CAD build for the part. Positions are in the model's coordinates, mm. Give positions to 0.01 mm unless a question says otherwise; leave off trailing zeros. Order: outer loops, then holes, each group sorted by start corner. A loop starts at its lowest first (then second) coordinate and runs counter-clockwise, first axis right, second up. Notation, with made-up numbers: (-27.75, 43) -> (-22.75, 43) arc R21 ccw to (-22.75, 62) -> close; hole circle Ø3 at (23, -10). An arc over 180 degrees is marked (long way). Use one line per item in the form item = value. Start each with the question number.
1) Drop flat-ended pins along their axis: P1, Ø1, axis at x = 0, z = -3.5, coming from the -Y side; P2, Ø2, axis at y = -1, z = 1, coming from the +X side; P3, Ø1.5, axis at x = -1, y = -1.5, coming from the +Z side; P4, Ø2, axis at x = -1, y = 2.5, coming from the -Z side. Give the stop position or say it passes through.
2) Probe line 1 (Y direction, x = 1.45, z = -0.5); line 2 (Y direction, x = 0.25, z = -0.75); line 3 (Z direction, x = -0.8, y = -0.25). List the from-to ranges inside material, lowest first.
3) Mould opens along Z. For faces 1 (the face through (1.86, -2, 3)), 2 (the face through (1.461, -0.963, -4.334)), 3 (the face through (0, -3, 0)) say: pulls with the +Z half, pulls with the -Z half, needs draft (parallel to the pull), parting line crosses it, or undercut.
4) Cut at C-C, the plane x = -0.55. Give the cut face in (y, z).
5) Cut at A-A, the plane z = 0. Give the cut face in (x, y).
from build123d import *

# Parameters (mm, degrees)
SCALE1_SCALE = 1.2
SCALE2_SCALE = 0.1


with BuildPart() as part:
    # Sketch1 → Revolve1 (revolve)
    with BuildSketch(Plane.XY):
        with BuildLine():
            Line((-13.4, 25), (13.4, 25))
            ThreePointArc((13.4, 25), (14.88492424, 25.61507576), (15.5, 27.1))
            Line((15.5, 27.1), (15.5, 37))
            Line((15.5, 37), (8.94427191, 37))
            ThreePointArc((8.94427191, 37), (0, 33), (-8.94427191, 37))
            Line((-8.94427191, 37), (-15.5, 37))
            Line((-15.5, 37), (-15.5, 27.1))
            ThreePointArc((-15.5, 27.1), (-14.88492424, 25.61507576), (-13.4, 25))
        make_face()
    revolve(axis=Axis((-24.473684211, 0, 0), (1, 0, 0)))


with BuildPart() as part_1:
    # Scale1: scaled about (0, 0, 0)
    add(part.part.scale(SCALE1_SCALE))


with BuildPart() as part_2:
    # Scale2: scaled about (0, 0, 0)
    add(part_1.part.scale(SCALE2_SCALE))


solid = part_2.part
Result:
q1.P1 = -2.58
q1.P2 = through
q1.P3 = 4.38
q1.P4 = -4.18
q2.line_1 = -4.41 to -2.96, 2.96 to 4.41
q2.line_2 = -3.91 to -2.9, 2.9 to 3.91
q2.line_3 = -4.2 to -2.99, 2.99 to 4.2
q3.face_1 = needs draft
q3.face_2 = parting line crosses it
q3.face_3 = undercut
q4.outline = circle Ø8.14 at (0, 0); hole circle Ø6 at (0, 0)
q5.outline = (-1.86, -4.44) -> (-1.07, -4.44) arc R1.44 cw to (1.07, -4.44) -> (1.86, -4.44) -> (1.86, -3.25) arc R0.25 ccw to (1.61, -3) -> (-1.61, -3) arc R0.25 ccw to (-1.86, -3.25) -> close; (-1.86, 3.25) arc R0.25 ccw to (-1.61, 3) -> (1.61, 3) arc R0.25 ccw to (1.86, 3.25) -> (1.86, 4.44) -> (1.07, 4.44) arc R1.44 cw to (-1.07, 4.44) -> (-1.86, 4.44) -> close
